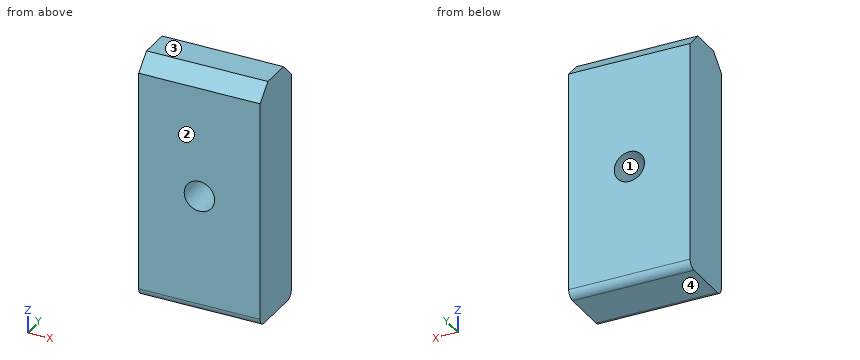
```python
from build123d import *

# Parameters (mm, degrees)
F0_W     = 1.1063814163
F0_H     = 17.7862383425
F1_DEPTH = 200
F2_SIZE  = 50
F3_R     = 25
F5_D     = 100


with BuildPart() as f1:
    # F0 (on Front) → F1 (new body)
    with BuildSketch(Plane.XZ):
        with Locations((170.4081445932, 8.8931191713)):
            Rectangle(F0_W, F0_H)
        Polygon((0, 800), (0, 0), (169.8549538851, 0), (169.8549538851, 17.7862383425), (170.9613353014, 17.7862383425), (170.9613353014, 0), (400, 0), (400, 800), align=None)
    extrude(amount=F1_DEPTH)

    # F2
    f2_edges = [f1.edges().sort_by_distance(p)[0] for p in [
        (200, -200, 800),
        (200, 0, 800),
    ]]
    chamfer(f2_edges, length=F2_SIZE)

    # F3
    f3_edges = [f1.edges().sort_by_distance(p)[0] for p in [
        (200, -200, 0),
        (200, 0, 0),
    ]]
    fillet(f3_edges, radius=F3_R)

    # F5 (through all)
    with Locations(Plane.XZ.offset(200)):
        with Locations((200, 387.5)):
            Hole(F5_D / 2)


solid = f1.part
```
Part model, mm, in its own coordinate system. Face numbers are marked on the shaded views. Round coordinates to 2 decimals unless told otherwise and drop trailing zeros. Write each loop counter-clockwise with the first axis right and the second up, starting at its lowest first coordinate (ties: lowest second). Pieces come first, ordered by that corner, then holes.
Item 1: Cut at C-C, the plane y = -81. Give the cut face in (x, z).
Results:
outline: (0, 0) - (400, 0) - (400, 800) - (0, 800) - close; hole circle Ø100 at (200, 387.5)
Item 2: Drop flat-ended pins along their axis: pin 1 Ø1.5 at (x, y) = (136.5, -167) entering from +Z; pin 2 Ø5 at (y, z) = (-80.5, 534) entering from -X. Give the stop position or say it passes through.
Results:
pin 1: stops at z = 783.75
pin 2: stops at x = 0
Item 3: Cut at D-D, the plane x = 315.5. Give the cut face in (y, z), plus the area to 3 significant figures.
Results:
outline: (-200, 25) arc R25 ccw to (-175, 0) - (-25, 0) arc R25 ccw to (0, 25) - (0, 750) - (-50, 800) - (-150, 800) - (-200, 750) - close
area: 157,000 mm2
Item 4: Two-plate mould, pull along Z, no slides. Class the marked faces 1, 2, 3 and 4: +Z half, -Z half, draft (parallel to the pull), parting line (faces both ways), or undercut.
Results:
face 1: undercut
face 2: draft
face 3: +Z half
face 4: -Z half
Item 5: Cut at A-A, the plane z = 387.5. Give the cut face in (x, y), plus the area to 3 significant figures.
Results:
outline: (0, -200) - (150, -200) - (150, 0) - (0, 0) - close; (250, -200) - (400, -200) - (400, 0) - (250, 0) - close
area: 60,000 mm2
Item 6: Probe L1, parallel to Z at x = 200, y = -104; L2, parallel to X at y = -140, z = 387; L3, parallel to X at y = -83.5, z = 361. List the from-to ranges inside material, lowest first.
Results:
L1: z = 0 to 337.5, 437.5 to 800
L2: x = 0 to 150, 250 to 400
L3: x = 0 to 157.6, 242.4 to 400
Item 7: Cut at B-B, the plane x = 200. Give the cut face in (y, z), plus the area to 3 significant figures.
Results:
outline: (-200, 25) arc R25 ccw to (-175, 0) - (-25, 0) arc R25 ccw to (0, 25) - (0, 337.5) - (-200, 337.5) - close; (-200, 437.5) - (0, 437.5) - (0, 750) - (-50, 800) - (-150, 800) - (-200, 750) - close
area: 137,000 mm2
